from build123d import *

# Parameters (mm, degrees)
F0_R     = 11.049
F1_DEPTH = 7.62


with BuildPart() as f1:
    # F0 (on Top) → F1 (new body)
    with BuildSketch(Plane.XY):
        with BuildLine():
            ThreePointArc((0.039662, 21.40109), (6.089549, 31.577889), (17.220307, 35.612065))
            ThreePointArc((17.220307, 35.612065), (-1.561389, 31.350671), (-13.725973, 16.41968))
            ThreePointArc((-13.725973, 16.41968), (-15.633011, 28.104353), (-9.699474, 38.349425))
            ThreePointArc((-9.699474, 38.349425), (-21.347916, 23.012366), (-21.069072, 3.755319))
            ThreePointArc((-21.069072, 3.755319), (-30.040711, 11.480478), (-32.080763, 23.142662))
            ThreePointArc((-32.080763, 23.142662), (-31.145516, 3.906319), (-18.553719, -10.666197))
            ThreePointArc((-18.553719, -10.666197), (-30.392028, -10.51524), (-39.451107, -2.892809))
            ThreePointArc((-39.451107, -2.892809), (-26.369783, -17.027538), (-7.356874, -20.096881))
            ThreePointArc((-7.356874, -20.096881), (-16.522578, -27.590761), (-28.361839, -27.574703))
            ThreePointArc((-28.361839, -27.574703), (-9.255335, -29.994021), (7.282334, -20.124012))
            ThreePointArc((7.282334, -20.124012), (5.07797, -31.756257), (-4.001752, -39.354087))
            ThreePointArc((-4.001752, -39.354087), (12.189787, -28.925968), (18.514057, -10.734893))
            ThreePointArc((18.514057, -10.734893), (24.302479, -21.062648), (22.2308, -32.719256))
            ThreePointArc((22.2308, -32.719256), (27.931172, -14.323133), (21.082847, 3.677201))
            ThreePointArc((21.082847, 3.677201), (32.155589, -0.513592), (38.061313, -10.774722))
            ThreePointArc((38.061313, -10.774722), (30.603252, 6.981655), (13.786738, 16.368692))
            ThreePointArc((13.786738, 16.368692), (24.962741, 20.27578), (36.082515, 16.211425))
            ThreePointArc((36.082515, 16.211425), (18.95573, 25.019649), (0.039662, 21.40109))
        make_face()
        Circle(F0_R, mode=Mode.SUBTRACT)
    extrude(amount=F1_DEPTH)


solid = f1.part
The listing builds one solid part. Answer for the finished solid, in the listing's coordinates (mm). Round coordinates to 2 decimals unless told otherwise and drop trailing zeros. Order: outer loops, then holes, each group sorted by start corner. A loop starts at its lowest first (then second) coordinate and runs counter-clockwise, first axis right, second up. Notation, with made-up numbers: (-38, 14) -> (-33, 14) arc R13 ccw to (-33, 26) -> close; hole circle Ø6 at (7, -21). An arc over 180 degrees is marked (long way). One line per item, written item: value.
Item 1: For a pull along Y with two mould halves and no side action, classify faces 1 (the cylindrical face through (-30.233, -10.573, 3.757)), 2 (the cylindrical face through (-9.52, -30.05, 3.76)), 3 (the flat face through (7, -9, 7.62)) as released by +Y, released by -Y, zero draft, split by the parting line, or undercut.
Taken from the geometry:
face 1: undercut
face 2: undercut
face 3: zero draft
Item 2: Find section B-B, the plane z = 3.25. Give the vertices of the cut face in (x, y).
Taken from the geometry:
outline: (-39.45, -2.89) arc R29.54 ccw to (-7.36, -20.1) arc R17.58 cw to (-28.36, -27.57) arc R29.54 ccw to (7.28, -20.12) arc R17.58 cw to (-4, -39.35) arc R29.54 ccw to (18.51, -10.73) arc R17.58 cw to (22.23, -32.72) arc R29.54 ccw to (21.08, 3.68) arc R17.58 cw to (38.06, -10.77) arc R29.54 ccw to (13.79, 16.37) arc R17.58 cw to (36.08, 16.21) arc R29.54 ccw to (0.04, 21.4) arc R17.58 cw to (17.22, 35.61) arc R29.54 ccw to (-13.73, 16.42) arc R17.58 cw to (-9.7, 38.35) arc R29.54 ccw to (-21.07, 3.76) arc R17.58 cw to (-32.08, 23.14) arc R29.54 ccw to (-18.55, -10.67) arc R17.58 cw to start; hole circle Ø22.1 at (0, 0)
Item 3: Find section D-D, the plane y = -15.5. Give the vertices of the cut face in (x, z).
Taken from the geometry:
outline: (-28.91, 0) -> (18.11, 0) -> (18.11, 7.62) -> (-28.91, 7.62) -> close; (22.36, 0) -> (27.94, 0) -> (27.94, 7.62) -> (22.36, 7.62) -> close
Item 4: Find section C-C, the plane x = -17.5. Give the vertices of the cut face in (y, z).
Taken from the geometry:
outline: (-30.54, 0) -> (-27.91, 0) -> (-27.91, 7.62) -> (-30.54, 7.62) -> close; (-20.09, 0) -> (30.71, 0) -> (30.71, 7.62) -> (-20.09, 7.62) -> close
Item 5: Straight lines are drawn through the part: L1, parallel to X at y = -2.5, z = 5.5; L2, parallel to Y at x = 0, z = 1.75; L3, parallel to X at y = 18, z = 1. For each, find the intervals that lie inside material, in ascending order.
Taken from the geometry:
L1: x = -27.61 to -10.76, 10.76 to 25.05, 34.14 to 36.3
L2: y = -38.07 to -37.26, -26.35 to -11.05, 11.05 to 32.25
L3: x = -33.09 to -32.2, -22.52 to -14.5, -13.09 to 16.19, 33.49 to 34.21
Item 6: Find section A-A, the plane y = -25. Give the vertices of the cut face in (x, z).
Taken from the geometry:
outline: (-11.75, 0) -> (2.03, 0) -> (2.03, 7.62) -> (-11.75, 7.62) -> close; (7.37, 0) -> (14.8, 0) -> (14.8, 7.62) -> (7.37, 7.62) -> close; (24.52, 0) -> (26.29, 0) -> (26.29, 7.62) -> (24.52, 7.62) -> close
Item 7: Given P1, Ø4, axis at x = 27, y = -1.5, coming from the -Z side, flat-ended and moving along its own axis, determine where the tip first touches the part or whether it passes through.
Taken from the geometry:
P1: passes through
